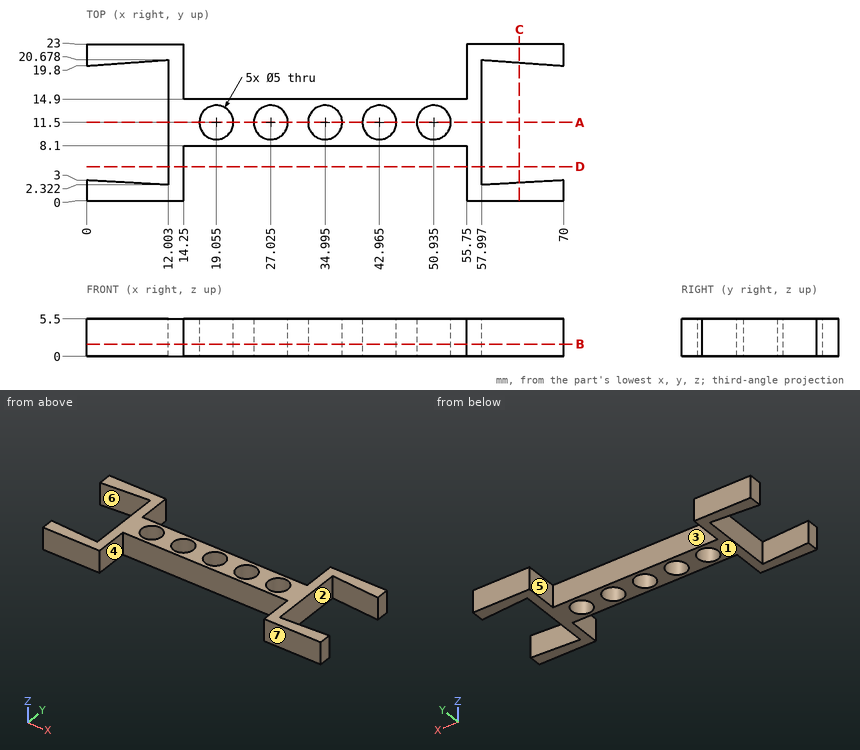
Input: dimensioned drawing with shaded views. Units: mm. Origin: part minimum x, y, z. A direction names the side the tool comes from. Coordinates: 2 decimals unless noted, no trailing zeros. Order: outer loops, then holes, each group sorted by start corner. A loop starts at its lowest first (then second) coordinate and runs counter-clockwise, first axis right, second up. Notation, with made-up numbers: (80, 30) - (88, 30) arc R3 ccw to (88, 35) - close; hole circle Ø2 at (1, -23). An arc over 180 degrees is marked (long way). One line per item, written item: value.
1) Ray query, line 1 (X direction, y = 2, z = 4.2); line 2 (X direction, y = 16.5, z = 2.9); line 3 (Y direction, x = 55.5, z = 5.2). Return the intervals inside material, ascending. Write a range as [from, to].
Computed values:
line 1: x = [0, 14.25], [55.75, 70]
line 2: x = [12, 14.25], [55.75, 58]
line 3: y = [8.1, 14.9]
2) Cut plane A-A on y = 11.5. Output: boundary loops of the cut face in (x, z) (1 decimal).
Computed values:
outline: (12, 0) - (16.6, 0) - (16.6, 5.5) - (12, 5.5) - close; (21.6, 0) - (24.5, 0) - (24.5, 5.5) - (21.6, 5.5) - close; (29.5, 0) - (32.5, 0) - (32.5, 5.5) - (29.5, 5.5) - close; (37.5, 0) - (40.5, 0) - (40.5, 5.5) - (37.5, 5.5) - close; (45.5, 0) - (48.4, 0) - (48.4, 5.5) - (45.5, 5.5) - close; (53.4, 0) - (58, 0) - (58, 5.5) - (53.4, 5.5) - close
3) Cut plane C-C on x = 63.5. Output: boundary loops of the cut face in (y, z) (1 decimal).
Computed values:
outline: (0, 0) - (2.6, 0) - (2.6, 5.5) - (0, 5.5) - close; (20.3, 0) - (23, 0) - (23, 5.5) - (20.3, 5.5) - close
4) Cut plane D-D on y = 5. Output: boundary loops of the cut face in (x, z), plus the area to 3 significant figures.
Computed values:
outline: (12, 0) - (14.25, 0) - (14.25, 5.5) - (12, 5.5) - close; (55.75, 0) - (58, 0) - (58, 5.5) - (55.75, 5.5) - close
area: 24.7 mm^2
5) Reachability of the marked faces 4, 5, 6 and 7 from +Z, -Z, +X, -X, +Y, -Y: full face, straight path, thin tool, end or side. Return the list, or none.
Computed values:
face 4: +Z, -Z, -Y
face 5: +Z, -Z, +Y
face 6: +Z, -Z
face 7: +Z, -Z, +X, -X, -Y
6) Cut plane B-B on z = 1.8. State how many separate pieces and enclosed holes the cut face has.
Computed values:
separate pieces: 1
enclosed holes: 5
7) Mould query, pull axis Y, two halves, no side actions, for the marked faces 1, 2 and 3. Classes: released by +Y, released by -Y, zero draft, split by the parting line, or undercut.
Computed values:
face 1: zero draft
face 2: undercut
face 3: released by +Y
8) Contact query for flat-ended pins moving along their axis: pin 1 (4 mm diameter, centred on x = 19.055, y = 11.5, fed in from +Z); pin 2 (3 mm diameter, centred on x = 34.5, z = 4, fed in from +Y); pin 3 (1.6 mm diameter, centred on y = 15.5, z = 4, fed in from +X); pin 4 (1.6 mm diameter, centred on y = 17, z = 3.5, fed in from -X). Output: stop coordinate, or through.
Computed values:
pin 1: passes through
pin 2: stops at y = 14.9
pin 3: stops at x = 58
pin 4: stops at x = 12
